Part model, mm, in its own coordinate system. Face numbers are marked on the shaded views. A direction names the side the tool comes from. Coordinates: 2 decimals unless noted, no trailing zeros. Loops run counter-clockwise (first coordinate to the right, second up) from the corner with the lowest first, then second, coordinate; pieces in that order, holes last.
Solid Edge part; units mm, degrees
sketch "Sketch1" plane through (0, 0, 0) normal (0, 0, 1) x (1, 0, 0)
  line L0 (-14, -6) -> (14, -6)
  arc A0 (14, -6) -> (16, -4) centre (14, -4) ccw
  line L1 (16, -4) -> (16, 4)
  arc A1 (16, 4) -> (14, 6) centre (14, 4) ccw
  line L2 (14, 6) -> (-14, 6)
  arc A2 (-14, 6) -> (-16, 4) centre (-14, 4) ccw
  line L3 (-16, 4) -> (-16, -4)
  arc A3 (-14, -6) -> (-16, -4) centre (-14, -4) cw
extrude "Protrusion1" add sketch "Sketch1" along normal blind 2
sketch "Sketch2" plane through (0, 0, 2) normal (0, 0, 1) x (1, 0, 0)
  line L0 (-15.5, -7.5) -> (15.5, -7.5)
  arc A0 (15.5, -7.5) -> (17.5, -5.5) centre (15.5, -5.5) ccw
  line L1 (17.5, -5.5) -> (17.5, 5.5)
  arc A1 (17.5, 5.5) -> (15.5, 7.5) centre (15.5, 5.5) ccw
  line L2 (15.5, 7.5) -> (-15.5, 7.5)
  arc A2 (-15.5, 7.5) -> (-17.5, 5.5) centre (-15.5, 5.5) ccw
  line L3 (-17.5, 5.5) -> (-17.5, -5.5)
  arc A3 (-15.5, -7.5) -> (-17.5, -5.5) centre (-15.5, -5.5) cw
extrude "ExtrudedProtrusion_2" add sketch "Sketch2" along normal blind 2
sketch "Sketch3" plane through (0, 0, 0) normal (0, 0, -1) x (1, 0, 0)
  circle A0 centre (-11, 0) radius 2
  circle A1 centre (11, 0) radius 2
  dimension "D1" = 11
extrude "ExtrudedCutout_1" cut sketch "Sketch3" against normal blind 7.258
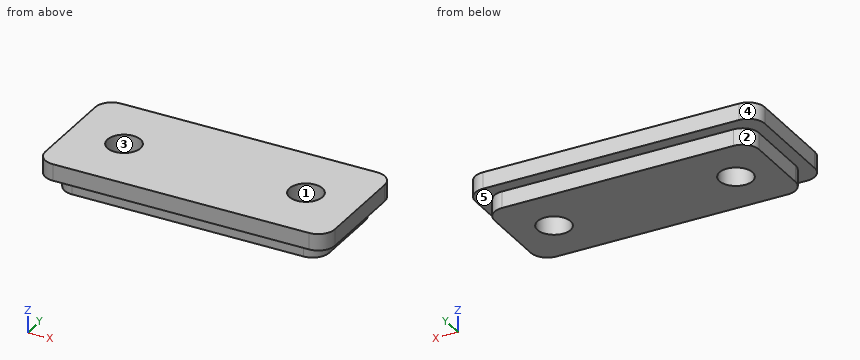
Q1. Probe line 1 (X direction, y = 0, z = 2.7); line 2 (X direction, y = 0, z = 1.5); line 3 (Y direction, x = -11, z = 1.25). List the from-to ranges inside material, lowest first.
Q2. Saw through at A-A (x = -11). List the corners of the cut face in (y, z), plus the area to 3 significant figures.
Q3. Saw through at D-D (y = 2.75). List the corners of the cut face in (x, z), plus the area to 3 significant figures.
Q4. Mould opens along X. For the marked faces 3, 4 and 5 say: released by +X, released by -X, zero draft, split by the parting line, or undercut.
Q5. Saw through at C-C (y = 0). List the corners of the cut face in (x, z), plus the area to 3 significant figures.
Q6. Saw through at B-B (z = 0.5). List the corners of the cut face in (x, y), plus the area to 3 significant figures.
Q7. Tool access for the marked faces 1 and 2: list every direction of +Z, -Z, +X, -X, +Y, -Y with a clear straight run to the whole face (end or side of a thin tool).
Q8. Drop flat-ended pins along their axis: P1, Ø0.6, axis at x = 3, z = 1, coming from the -Y side; P2, Ø1.6, axis at y = -0.5, z = 1, coming from the +X side; P3, Ø2.5, axis at x = -11, y = 0, coming from the +Z side; P4, Ø0.6, axis at x = -4, z = 0.5, coming from the +Y side. Give the stop position or say it passes through.
Checked values:
1. line 1: x = -17.5 to -13, -9 to 9, 13 to 17.5
1. line 2: x = -16 to -13, -9 to 9, 13 to 16
1. line 3: y = -6 to -2, 2 to 6
2. outline: (-7.5, 2) - (-6, 2) - (-6, 0) - (-2, 0) - (-2, 4) - (-7.5, 4) - close; (2, 0) - (6, 0) - (6, 2) - (7.5, 2) - (7.5, 4) - (2, 4) - close
2. area: 38.0 mm2
3. outline: (-17.5, 2) - (-16, 2) - (-16, 0) - (16, 0) - (16, 2) - (17.5, 2) - (17.5, 4) - (-17.5, 4) - close
3. area: 134 mm2
4. face 3: undercut
4. face 4: released by -X
4. face 5: zero draft
5. outline: (-17.5, 2) - (-16, 2) - (-16, 0) - (-13, 0) - (-13, 4) - (-17.5, 4) - close; (-9, 0) - (9, 0) - (9, 4) - (-9, 4) - close; (13, 0) - (16, 0) - (16, 2) - (17.5, 2) - (17.5, 4) - (13, 4) - close
5. area: 102 mm2
6. outline: (-16, -4) arc R2 ccw to (-14, -6) - (14, -6) arc R2 ccw to (16, -4) - (16, 4) arc R2 ccw to (14, 6) - (-14, 6) arc R2 ccw to (-16, 4) - close; hole circle Ø4 at (-11, 0); hole circle Ø4 at (11, 0)
6. area: 355 mm2
7. face 1: +Z, -Z
7. face 2: -Z, -X, +Y
8. P1: stops at y = -6
8. P2: stops at x = 16
8. P3: passes through
8. P4: stops at y = 6
